from build123d import *

# Parameters (mm, degrees)
ESQUISSE1_R                  = 50
BOSS_EXTRU_1_DEPTH           = 71
COQUE1_T                     = -8
ESQUISSE2_R                  = 42
ESQUISSE2_R_2                = 1.625
ENL_V_MAT_EXTRU_4_DEPTH      = 71
ESQUISSE2_5_R                = 42
ESQUISSE2_5_R_2              = 1.625
BOSS_EXTRU_4_DEPTH           = 52
ESQUISSE2_6_R                = 42
ESQUISSE2_6_R_2              = 1.625
ENL_V_MAT_EXTRU_5_DEPTH      = 50
ENL_V_MAT_EXTRU_6_REACH      = 102.205
ESQUISSE2_7_R                = 1.625
ENL_V_MAT_EXTRU_7_REACH      = 134.442
ENL_V_MAT_EXTRU_7_END_RADIUS = 42
ESQUISSE9_W                  = 8
ESQUISSE9_H                  = 20
ESQUISSE14_R                 = 1.75
BOSS_EXTRU_6_DEPTH           = 2
CONG_1_R                     = 2
CONG_2_R                     = 3.5


with BuildPart() as part:
    # Esquisse1 → Boss.-Extru.1 (new body)
    with BuildSketch(Plane.XY):
        Circle(ESQUISSE1_R)
    extrude(amount=BOSS_EXTRU_1_DEPTH)

    # Coque1
    coque1_openings = [part.faces().sort_by_distance(p)[0] for p in [
        (0, 0, 71),
    ]]
    offset(amount=COQUE1_T, openings=coque1_openings, kind=Kind.INTERSECTION)

    # Esquisse2 → Enl_v. mat.-Extru.4 (cut)
    with BuildSketch(Plane.XY.offset(71)):
        Circle(ESQUISSE2_R)
        with Locations((-21.75, -21.75)):
            Circle(ESQUISSE2_R_2, mode=Mode.SUBTRACT)
        with Locations((21.75, -21.75)):
            Circle(ESQUISSE2_R_2, mode=Mode.SUBTRACT)
        with Locations((21.75, 21.75)):
            Circle(ESQUISSE2_R_2, mode=Mode.SUBTRACT)
        with Locations((-21.75, 21.75)):
            Circle(ESQUISSE2_R_2, mode=Mode.SUBTRACT)
        with Locations((-21.75, 21.75)):
            Circle(ESQUISSE2_R_2)
        with Locations((-21.75, -21.75)):
            Circle(ESQUISSE2_R_2)
        with Locations((21.75, -21.75)):
            Circle(ESQUISSE2_R_2)
        with Locations((21.75, 21.75)):
            Circle(ESQUISSE2_R_2)
    extrude(amount=-ENL_V_MAT_EXTRU_4_DEPTH, mode=Mode.SUBTRACT)

    # Esquisse2_5 → Boss.-Extru.4 (add)
    with BuildSketch(Plane.XY.offset(71)):
        Circle(ESQUISSE2_5_R)
        with Locations((-21.75, -21.75)):
            Circle(ESQUISSE2_5_R_2, mode=Mode.SUBTRACT)
        with Locations((21.75, -21.75)):
            Circle(ESQUISSE2_5_R_2, mode=Mode.SUBTRACT)
        with Locations((21.75, 21.75)):
            Circle(ESQUISSE2_5_R_2, mode=Mode.SUBTRACT)
        with Locations((-21.75, 21.75)):
            Circle(ESQUISSE2_5_R_2, mode=Mode.SUBTRACT)
        with Locations((-21.75, 21.75)):
            Circle(ESQUISSE2_5_R_2)
        with Locations((21.75, 21.75)):
            Circle(ESQUISSE2_5_R_2)
        with Locations((21.75, -21.75)):
            Circle(ESQUISSE2_5_R_2)
        with Locations((-21.75, -21.75)):
            Circle(ESQUISSE2_5_R_2)
    extrude(amount=-BOSS_EXTRU_4_DEPTH)

    # Esquisse2_6 → Enl_v. mat.-Extru.5 (cut)
    with BuildSketch(Plane.XY.offset(71)):
        Circle(ESQUISSE2_6_R)
        with Locations((-21.75, 21.75)):
            Circle(ESQUISSE2_6_R_2, mode=Mode.SUBTRACT)
        with Locations((21.75, 21.75)):
            Circle(ESQUISSE2_6_R_2, mode=Mode.SUBTRACT)
        with Locations((21.75, -21.75)):
            Circle(ESQUISSE2_6_R_2, mode=Mode.SUBTRACT)
        with Locations((-21.75, -21.75)):
            Circle(ESQUISSE2_6_R_2, mode=Mode.SUBTRACT)
    extrude(amount=-ENL_V_MAT_EXTRU_5_DEPTH, mode=Mode.SUBTRACT)

    # Esquisse2_7 → Enl_v. mat.-Extru.6 (cut, up to next)
    with BuildSketch(Plane.XY.offset(71), mode=Mode.PRIVATE) as enl_v_mat_extru_6_sk1:
        with Locations((-21.75, 21.75)):
            Circle(ESQUISSE2_7_R)
    enl_v_mat_extru_6_tool1 = extrude(enl_v_mat_extru_6_sk1.sketch, amount=-ENL_V_MAT_EXTRU_6_REACH, mode=Mode.PRIVATE) & part.part
    # Esquisse2_7 → Enl_v. mat.-Extru.6 (cut, up to next)
    with BuildSketch(Plane.XY.offset(71), mode=Mode.PRIVATE) as enl_v_mat_extru_6_sk2:
        with Locations((21.75, 21.75)):
            Circle(ESQUISSE2_7_R)
    enl_v_mat_extru_6_tool2 = extrude(enl_v_mat_extru_6_sk2.sketch, amount=-ENL_V_MAT_EXTRU_6_REACH, mode=Mode.PRIVATE) & part.part
    # Esquisse2_7 → Enl_v. mat.-Extru.6 (cut, up to next)
    with BuildSketch(Plane.XY.offset(71), mode=Mode.PRIVATE) as enl_v_mat_extru_6_sk3:
        with Locations((21.75, -21.75)):
            Circle(ESQUISSE2_7_R)
    enl_v_mat_extru_6_tool3 = extrude(enl_v_mat_extru_6_sk3.sketch, amount=-ENL_V_MAT_EXTRU_6_REACH, mode=Mode.PRIVATE) & part.part
    # Esquisse2_7 → Enl_v. mat.-Extru.6 (cut, up to next)
    with BuildSketch(Plane.XY.offset(71), mode=Mode.PRIVATE) as enl_v_mat_extru_6_sk4:
        with Locations((-21.75, -21.75)):
            Circle(ESQUISSE2_7_R)
    enl_v_mat_extru_6_tool4 = extrude(enl_v_mat_extru_6_sk4.sketch, amount=-ENL_V_MAT_EXTRU_6_REACH, mode=Mode.PRIVATE) & part.part
    add(enl_v_mat_extru_6_tool1.solids().sort_by_distance((-21.75, 21.75, 71))[0], mode=Mode.SUBTRACT)
    add(enl_v_mat_extru_6_tool2.solids().sort_by_distance((21.75, 21.75, 71))[0], mode=Mode.SUBTRACT)
    add(enl_v_mat_extru_6_tool3.solids().sort_by_distance((21.75, -21.75, 71))[0], mode=Mode.SUBTRACT)
    add(enl_v_mat_extru_6_tool4.solids().sort_by_distance((-21.75, -21.75, 71))[0], mode=Mode.SUBTRACT)

    # Enl_v. mat.-Extru.7: up to this cylinder (the profile starts outside it)
    enl_v_mat_extru_7_end = Plane(origin=(0, 0, 15), z_dir=(0, 0, -1)) * Cylinder(ENL_V_MAT_EXTRU_7_END_RADIUS, 353.884, mode=Mode.PRIVATE)
    # Esquisse9 → Enl_v. mat.-Extru.7 (cut, up to the surface)
    with BuildSketch(Plane(origin=(50, 0, 0), x_dir=(0, 0, -1), z_dir=(1, 0, 0)), mode=Mode.PRIVATE) as enl_v_mat_extru_7_sk1:
        with Locations((-15, 0)):
            Rectangle(ESQUISSE9_W, ESQUISSE9_H)
    enl_v_mat_extru_7_tool1 = extrude(enl_v_mat_extru_7_sk1.sketch, amount=-ENL_V_MAT_EXTRU_7_REACH, mode=Mode.PRIVATE) - enl_v_mat_extru_7_end
    add(enl_v_mat_extru_7_tool1.solids().sort_by_distance((50, 0, 15))[0], mode=Mode.SUBTRACT)

    # Esquisse14 → Boss.-Extru.6 (add)
    with BuildSketch(Plane.XY.offset(65)):
        with BuildLine():
            Line((49.749371855, 5), (57.749371855, 5))
            Line((57.749371855, 5), (57.749371855, 13))
            Line((57.749371855, 13), (48.280430818, 13))
            ThreePointArc((48.280430818, 13), (49.177846161, 9.029919542), (49.749371855, 5))
        make_face()
        with Locations((53.749371855, 9)):
            Circle(ESQUISSE14_R, mode=Mode.SUBTRACT)
    boss_extru_6 = extrude(amount=-BOSS_EXTRU_6_DEPTH)

    # Sym_trie1: Boss.-Extru.6 across plane
    add(boss_extru_6.mirror(Plane(origin=(0, 0, 0), x_dir=(0, 0, 1), z_dir=(1, 0, 0))))

    # Cong_1
    cong_1_edges = [part.edges().sort_by_distance(p)[0] for p in [
        (49.749371855, 5, 64),
        (48.280430818, 13, 64),
        (49.177846161, 9.029919542, 63),
        (-49.177846161, 9.029919542, 63),
        (-48.280430818, 13, 64),
        (-49.749371855, 5, 64),
    ]]
    fillet(cong_1_edges, radius=CONG_1_R)

    # Cong_2
    cong_2_edges = [part.edges().sort_by_distance(p)[0] for p in [
        (57.749371855, 13, 64),
        (57.749371855, 5, 64),
        (-57.749371855, 5, 64),
        (-57.749371855, 13, 64),
    ]]
    fillet(cong_2_edges, radius=CONG_2_R)


solid = part.part
Read the model definition and answer for the solid it produces. Units are mm, in the model's axes. A direction names the side the tool comes from. Coordinates: 2 decimals unless noted, no trailing zeros. Loops run counter-clockwise (first coordinate to the right, second up) from the corner with the lowest first, then second, coordinate; pieces in that order, holes last. Notation, with made-up numbers: (49.25, 83) - (105.25, 83) arc R35 cw to (105.25, 122) - close; hole circle Ø1 at (74.25, 60). An arc over 180 degrees is marked (long way). Answer in a Markdown table with one row per item.
Q1. Find section D-D on z = 66.5. Write down the section's boundary in (x, y), plus the area to 3 significant figures.
Here are the results:
| item | result |
|---|---|
| outline | circle Ø100 at (0, 0); hole circle Ø84 at (0, 0) |
| area | 2,310 mm^2 |
Q2. The mould has two halves that part along X. Classify faces 6 (the flat face through (-56, 9, 63)), 7 (the cylindrical face through (23.25, 21.13, 20.01)), 8 (the cylindrical face through (56.75, 11.95, 63.99)): pulls with the +X half, pulls with the -X half, needs draft (parallel to the pull), parting line crosses it, or undercut.
Here are the results:
| item | result |
|---|---|
| face 6 | needs draft |
| face 7 | undercut |
| face 8 | pulls with the +X half |
Q3. Given P1, Ø3, axis at x = -53.75, y = 9, coming from the -Z side; P2, Ø12, axis at y = -13, z = 30, coming from the -X side; P3, Ø3.5, axis at x = -21.75, y = -21.75, coming from the -Z side; P4, Ø3.5, axis at x = -21.75, y = 21.75, coming from the +Z side, each flat-ended and moving along its own axis, determine where each tip first touches the part or whether it passes through.
Here are the results:
| item | result |
|---|---|
| P1 | passes through |
| P2 | stops at x = -49.51 |
| P3 | stops at z = 19 |
| P4 | stops at z = 21 |
Q4. Straight lines are drawn through the part: line 1 along Y through (x, z) = (0, 14.25); line 2 along Z through (x, y) = (44, -8.5); line 3 along Y through (x, z) = (-21.75, 19.4) (3 decimals). For each, find the intervals that lie inside material, in ascending order. Write a range as [from, to].
Here are the results:
| item | result |
|---|---|
| line 1 | y = [-50, -42], [42, 50] |
| line 2 | z = [0, 11], [19, 71] |
| line 3 | y = [-45.022, -23.375], [-20.125, 20.125], [23.375, 45.022] |
Q5. Find section B-B on x = -21.75. Write down the section's boundary in (y, z) (3 decimals), plus the area to 3 significant figures.
Here are the results:
| item | result |
|---|---|
| outline | (-45.022, 0) - (-35.93, 0) - (-35.93, 19) - (-23.375, 19) - (-23.375, 21) - (-35.93, 21) - (-35.93, 71) - (-45.022, 71) - close; (-20.125, 19) - (20.125, 19) - (20.125, 21) - (-20.125, 21) - close; (23.375, 19) - (35.93, 19) - (35.93, 0) - (45.022, 0) - (45.022, 71) - (35.93, 71) - (35.93, 21) - (23.375, 21) - close |
| area | 1,420 mm^2 |
Q6. Find section A-A on y = 0. Write down the section's boundary in (x, z), plus the area to 3 significant figures.
Here are the results:
| item | result |
|---|---|
| outline | (-50, 0) - (-42, 0) - (-42, 19) - (50, 19) - (50, 71) - (42, 71) - (42, 21) - (-42, 21) - (-42, 71) - (-50, 71) - close; (42, 0) - (50, 0) - (50, 11) - (42, 11) - close |
| area | 1,240 mm^2 |
Q7. For faces 1 (the flat face through (45, 10, 15)), 2 (the flat face through (-1, 1, 21)), 3 (the flat face through (-51.6, 8.7, 65)), 4 (the cylindrical face through (19.38, -37.26, 9.63)), 5 (the flat face through (51.6, 8.7, 65)), determine the directions among +Z, -Z, +X, -X, +Y, -Y from which every point of the face is accessible in a straight line to the end or side of a thin tool.
Here are the results:
| item | result |
|---|---|
| face 1 | +X |
| face 2 | +Z |
| face 3 | +Z, -X, +Y |
| face 4 | -Z |
| face 5 | +Z, +X, +Y |
